from build123d import *

# Parameters (mm, degrees)
SKETCH1_W           = 20
SKETCH1_H           = 20
BOSS_EXTRUDE1_DEPTH = 3
SKETCH2_W           = 3
SKETCH2_H           = 20
BOSS_EXTRUDE2_DEPTH = 150
SKETCH3_W           = 17
SKETCH3_H           = 3
BOSS_EXTRUDE3_DEPTH = 150
SKETCH4_R           = 1.6
CUT_EXTRUDE1_DEPTH  = 3
SKETCH5_W           = 30
SKETCH5_H           = 17
BOSS_EXTRUDE4_DEPTH = 4
SKETCH6_W           = 30
SKETCH6_H           = 17
BOSS_EXTRUDE5_DEPTH = 4
SKETCH9_R           = 2.05
SKETCH9_R_2         = 2.1
CUT_EXTRUDE4_DEPTH  = 186.434844337
SKETCH10_R          = 4
CUT_EXTRUDE5_DEPTH  = 2.5
SKETCH11_W          = 30
SKETCH11_H          = 7
CUT_EXTRUDE6_DEPTH  = 3
CHAMFER2_SIZE       = 1
CHAMFER3_SIZE       = 3
SKETCH12_W          = 3.1
SKETCH12_H          = 17
CUT_EXTRUDE7_DEPTH  = 3
SKETCH13_R          = 1.65
CUT_EXTRUDE8_DEPTH  = 3
SKETCH14_R          = 3
CUT_EXTRUDE9_DEPTH  = 6


with BuildPart() as part:
    # Sketch1 → Boss-Extrude1 (new body)
    with BuildSketch(Plane(origin=(0, 0, 0), x_dir=(0, 0, -1), z_dir=(1, 0, 0))):
        with Locations((-98.245468701, -9.501201475)):
            Rectangle(SKETCH1_W, SKETCH1_H)
    extrude(amount=BOSS_EXTRUDE1_DEPTH)

    # Sketch2 → Boss-Extrude2 (add)
    with BuildSketch(Plane.ZY):
        with Locations((106.745468701, -9.501201475)):
            Rectangle(SKETCH2_W, SKETCH2_H)
    extrude(amount=BOSS_EXTRUDE2_DEPTH)

    # Sketch3 → Boss-Extrude3 (add)
    with BuildSketch(Plane.ZY):
        with Locations((96.745468701, -18.001201475)):
            Rectangle(SKETCH3_W, SKETCH3_H)
    extrude(amount=BOSS_EXTRUDE3_DEPTH)

    # Sketch4 → Cut-Extrude1 (cut)
    with BuildSketch(Plane(origin=(3, 0, 0), x_dir=(0, 0, -1), z_dir=(1, 0, 0))):
        with Locations((-101.245468701, -4.501201475)):
            Circle(SKETCH4_R)
        with Locations((-92.245468701, -4.501201475)):
            Circle(SKETCH4_R)
        with Locations((-92.245468701, -12.501201475)):
            Circle(SKETCH4_R)
        with Locations((-101.245468701, -12.501201475)):
            Circle(SKETCH4_R)
    extrude(amount=-CUT_EXTRUDE1_DEPTH, mode=Mode.SUBTRACT)

    # Sketch5 → Boss-Extrude4 (add)
    with BuildSketch(Plane(origin=(0, -16.501201475, 0), x_dir=(1, 0, 0), z_dir=(0, 1, 0))):
        with Locations((-135, -96.745468701)):
            Rectangle(SKETCH5_W, SKETCH5_H)
    extrude(amount=BOSS_EXTRUDE4_DEPTH)

    # Sketch6 → Boss-Extrude5 (add)
    with BuildSketch(Plane(origin=(0, -16.501201475, 0), x_dir=(1, 0, 0), z_dir=(0, 1, 0))):
        with Locations((-65, -96.745468701)):
            Rectangle(SKETCH6_W, SKETCH6_H)
    extrude(amount=BOSS_EXTRUDE5_DEPTH)

    # Sketch9 → Cut-Extrude4 (cut, through all)
    with BuildSketch(Plane(origin=(0, -12.501201475, 0), x_dir=(1, 0, 0), z_dir=(0, 1, 0))):
        with Locations(Location((-58, -96.745468701, 0), (0, 0, 270))):
            Circle(SKETCH9_R)
        with Locations(Location((-72, -96.745468701, 0), (0, 0, 270))):
            Circle(SKETCH9_R_2)
        with Locations(Location((-128, -96.745468701, 0), (0, 0, 270))):
            Circle(SKETCH9_R_2)
        with Locations(Location((-142, -96.745468701, 0), (0, 0, 270))):
            Circle(SKETCH9_R_2)
    extrude(amount=-CUT_EXTRUDE4_DEPTH, mode=Mode.SUBTRACT)

    # Sketch10 → Cut-Extrude5 (cut)
    with BuildSketch(Plane.XZ.offset(19.501201475)):
        with Locations(Location((-142, 96.745468701, 0), (0, 0, 270))):
            Circle(SKETCH10_R)
        with Locations(Location((-128, 96.745468701, 0), (0, 0, 270))):
            Circle(SKETCH10_R)
        with Locations(Location((-72, 96.745468701, 0), (0, 0, 270))):
            Circle(SKETCH10_R)
        with Locations(Location((-58, 96.745468701, 0), (0, 0, 270))):
            Circle(SKETCH10_R)
    extrude(amount=-CUT_EXTRUDE5_DEPTH, mode=Mode.SUBTRACT)

    # Sketch11 → Cut-Extrude6 (cut)
    with BuildSketch(Plane.XY.offset(108.245468701)):
        with Locations((-130, -6.001201475)):
            Rectangle(SKETCH11_W, SKETCH11_H)
    extrude(amount=-CUT_EXTRUDE6_DEPTH, mode=Mode.SUBTRACT)

    # Chamfer2
    chamfer2_edges = [part.edges().sort_by_distance(p)[0] for p in [
        (-145, -6.001201475, 105.245468701),
        (-130, -2.501201475, 105.245468701),
        (-115, -6.001201475, 105.245468701),
        (-130, -9.501201475, 105.245468701),
    ]]
    chamfer(chamfer2_edges, length=CHAMFER2_SIZE)

    # Chamfer3
    chamfer3_edges = [part.edges().sort_by_distance(p)[0] for p in [
        (-100, -16.501201475, 105.245468701),
        (-25, -16.501201475, 105.245468701),
    ]]
    chamfer(chamfer3_edges, length=CHAMFER3_SIZE)

    # Sketch12 → Cut-Extrude7 (cut)
    with BuildSketch(Plane(origin=(0, -16.501201475, 0), x_dir=(1, 0, 0), z_dir=(0, 1, 0))):
        with Locations((-118.45, -96.745468701)):
            Rectangle(SKETCH12_W, SKETCH12_H)
        with Locations((-81.55, -96.745468701)):
            Rectangle(SKETCH12_W, SKETCH12_H)
        with Locations((-48.45, -96.745468701)):
            Rectangle(SKETCH12_W, SKETCH12_H)
    extrude(amount=CUT_EXTRUDE7_DEPTH, mode=Mode.SUBTRACT)

    # Sketch13 → Cut-Extrude8 (cut)
    with BuildSketch(Plane(origin=(0, 0, 105.245468701), x_dir=(-1, 0, 0), z_dir=(0, 0, -1))):
        with Locations((100, -4.501201475)):
            Circle(SKETCH13_R)
        with Locations((100, -12.501201475)):
            Circle(SKETCH13_R)
    extrude(amount=-CUT_EXTRUDE8_DEPTH, mode=Mode.SUBTRACT)

    # Sketch14 → Cut-Extrude9 (cut)
    with BuildSketch(Plane(origin=(0, 0, 105.245468701), x_dir=(-1, 0, 0), z_dir=(0, 0, -1))):
        with Locations((100, -12.501201475)):
            Circle(SKETCH14_R)
    extrude(amount=CUT_EXTRUDE9_DEPTH, mode=Mode.SUBTRACT)


solid = part.part
Can you work these out from the model? Positions are in its coordinate system, mm. A direction names the side the tool comes from. Coordinates: 2 decimals unless noted, no trailing zeros. Write each loop counter-clockwise with the first axis right and the second up, starting at its lowest first coordinate (ties: lowest second). Pieces come first, ordered by that corner, then holes. Notation, with made-up numbers: (-14.75, 42.25) -> (3.25, 42.25) arc R5 ccw to (3.25, 47.25) -> close; hole circle Ø7 at (19.5, 86.5). An arc over 180 degrees is marked (long way). Write item = value, one per line.
(1) Imagine slicing it at A-A (x = -128). Please give me the cut outline in (y, z).
Verdict:
outline = (-19.5, 88.25) -> (-12.5, 88.25) -> (-12.5, 94.65) -> (-17, 94.65) -> (-17, 92.75) -> (-19.5, 92.75) -> close; (-19.5, 100.75) -> (-17, 100.75) -> (-17, 98.85) -> (-12.5, 98.85) -> (-12.5, 105.25) -> (-10.5, 105.25) -> (-9.5, 106.25) -> (-9.5, 108.25) -> (-19.5, 108.25) -> close; (-2.5, 106.25) -> (-1.5, 105.25) -> (0.5, 105.25) -> (0.5, 108.25) -> (-2.5, 108.25) -> close
(2) Thinking about a two-plate mould opening in Z: for faces 6 (the face through (-99.763, -15.689, 103.058)), 7 (the face through (-129.863, -14.72, 97.714)), 8 (the face through (-98.35, -4.43, 106.72)), which applies, +Z half, -Z half, draft (parallel to the pull), parting line (faces both ways), or undercut?
Verdict:
face_6 = -Z half
face_7 = undercut
face_8 = draft
(3) Imagine slicing it at C-C (x = -100). Please give me the cut outline in (y, z).
Verdict:
outline = (-19.5, 88.25) -> (-16.5, 88.25) -> (-16.5, 102.25) -> (-15.5, 103.25) -> (-15.5, 105.25) -> (-14.15, 105.25) -> (-14.15, 108.25) -> (-19.5, 108.25) -> close; (-10.85, 105.25) -> (-6.15, 105.25) -> (-6.15, 108.25) -> (-10.85, 108.25) -> close; (-2.85, 105.25) -> (0.5, 105.25) -> (0.5, 108.25) -> (-2.85, 108.25) -> close
(4) Imagine slicing it at B-B (y = -8.25). Please give me the cut outline in (x, z), and give its area (3 significant figures).
Verdict:
outline = (-150, 105.25) -> (-146, 105.25) -> (-145, 106.25) -> (-145, 108.25) -> (-150, 108.25) -> close; (-115, 106.25) -> (-114, 105.25) -> (0, 105.25) -> (0, 88.25) -> (3, 88.25) -> (3, 108.25) -> (-115, 108.25) -> close
area = 419 mm^2
(5) On a 3-axis mill with a long thin cutter (end or side, diameter ignored), from which of +Z, -Z, +X, -X, +Y, -Y can I reach the whole of each face in a straight line? I mean faces 1 (the face through (-73.53, -18.27, 93.05)), 2 (the face through (-100, -16.501, 95)), 3 (the face through (1.521, -12.431, 102.844)), 4 (the face through (-65, -12.501, 97)), 5 (the face through (1.521, -4.431, 93.844)). Say none if no direction works.
Verdict:
face_1 = -Y
face_2 = -Z, +Y
face_3 = +X
face_4 = -Z, -X, +Y
face_5 = +X, -X
(6) Imagine slicing it at D-D (x = -34). Please give me the cut outline in (y, z).
Verdict:
outline = (-19.5, 88.25) -> (-16.5, 88.25) -> (-16.5, 102.25) -> (-13.5, 105.25) -> (0.5, 105.25) -> (0.5, 108.25) -> (-19.5, 108.25) -> close
(7) If I drill on probe 1 along X at (y, z) = (-13, 99.25); probe 2 along Z at (x, y) = (-142, -14.8); probe 3 along X at (y, z) = (-17.25, 98.25), over which ranges is the centre line in solid material (lowest first)?
Verdict:
probe_1 = -150 to -120, -80 to -50, 0 to 3
probe_2 = 88.25 to 94.65, 98.85 to 108.25
probe_3 = -150 to -145.71, -138.29 to -131.71, -124.29 to -75.71, -68.29 to -61.71, -54.29 to 3
(8) For pin 1 (1.9 mm diameter, centred on y = -4.5, z = 101.25, fed in from +X); pin 2 (8.5 mm diameter, centred on x = -67.5, z = 96.5, fed in from +Y); pin 3 (3 mm diameter, centred on x = -112, z = 93.5, fed in from +Y); pin 4 (6.5 mm diameter, centred on x = -142, z = 96.75, fed in from -Y), each with a flat end and sliding along its axis, tell me the tip position at first contact or that it passes through.
Verdict:
pin_1 = through
pin_2 = -12.5
pin_3 = -16.5
pin_4 = -17
